```python
from build123d import *

# Parameters (mm, degrees)
F1_DEPTH = 25.4
F2_R     = 34.657222649
F3_DEPTH = 47.498
F4_R     = 5.08
F5_R     = 12.7
F6_DEPTH = 47.499
F7_R     = 5.08


with BuildPart() as f1:
    # F0 (on Top) → F1 (new body)
    with BuildSketch(Plane.XY):
        Polygon((43.3867163956, -75.1479971708), (43.3867163956, 75.1479971708), (-86.7734327912, 0), align=None)
    extrude(amount=F1_DEPTH)

    # F2 (on Top) → F3 (join)
    with BuildSketch(Plane.XY):
        Circle(F2_R)
    extrude(amount=F3_DEPTH)

    # F4
    f4_edges = [f1.edges().sort_by_distance(p)[0] for p in [
        (-34.657223, 0, 25.4),
        (-34.657223, 0, 47.498),
    ]]
    fillet(f4_edges, radius=F4_R)

    # F5 (on face) → F6 (cut, through all)
    with BuildSketch(Plane.XY.offset(47.498)):
        Circle(F5_R)
    extrude(amount=-F6_DEPTH, mode=Mode.SUBTRACT)

    # F7
    f7_edges = [f1.edges().sort_by_distance(p)[0] for p in [
        (43.386716, 0, 25.4),
        (-21.693358, -37.573999, 25.4),
        (-21.693358, 37.573999, 25.4),
        (43.386716, -75.147997, 12.7),
        (43.386716, 75.147997, 12.7),
        (-86.773433, 0, 12.7),
    ]]
    fillet(f7_edges, radius=F7_R)

    # F8 (on Right) → F9 (revolve)
    with BuildSketch(Plane.YZ):
        with BuildLine():
            Line((13.7427253649, 77.7795091271), (13.7427253649, 38.8897545636))
            add(Edge.make_bspline(
                [(13.7427253649, 77.7795091271), (19.7552349789, 72.2247905159), (30.7430265403, 62.0736067006), (63.7135258095, 65.9775971528), (32.8505351499, 49.2475903212), (13.7427253649, 38.8897545636)],
                knots=[0, 0, 0, 0, 0.3152034483, 0.5760306447, 1, 1, 1, 1], degree=3))
        make_face()
    revolve(axis=Axis((0, 0, 37.3068228364), (0, 0, 1)))


solid = f1.part
```
Model file for the job. Use its own axes, mm. A direction names the side the tool comes from. Give positions to 0.01 mm unless a question says otherwise; leave off trailing zeros. Loops run counter-clockwise (first coordinate to the right, second up) from the corner with the lowest first, then second, coordinate; pieces in that order, holes last. Notation, with made-up numbers: (-37, -18.75) -> (-27, -18.75) arc R23 cw to (-27, -1.75) -> close; hole circle Ø3 at (-38.75, -22). An arc over 180 degrees is marked (long way). Use CSV: the item, a comma, the result in double quotes. Start each with the question number.
1) Slice it at B-B on z = 28. Give the cut face in (x, y), plus the area to 3 significant figures.
2) Slice it at A-A on z = 18.5. Give the cut face in (x, y).
3) Wall check: line 1 (Y direction, x = 0, z = 33.5); line 2 (Z direction, x = -39, y = 11); line 3 (Y direction, x = 0, z = 17). Give the ranges that are in metal, low to high.
4) Mould opens along X. For faces 4 (the flat face through (9.1, -9.1, 47.498)), 5 (the flat face through (-51, 0, 25.4)), 6 (the cylindrical face through (12.038, 55.285, 23.951)), 7 (the cylindrical face through (-2.75, -12.4, 24.08)) say: released by +X, released by -X, zero draft, split by the parting line, or undercut.
5) Tool access for faces 1 (the flat face through (43.387, -1, 10)), 2 (the cylindrical face through (33.057, 10.41, 36.365)), 3 (the cylindrical face through (-54.57, 16.83, 23.95)): list every direction of +Z, -Z, +X, -X, +Y, -Y with a clear straight run to the whole face (end or side of a thin tool).
6) Flat gauge pins, fed straight in: pin 1 Ø2 at (x, z) = (-22.5, 37.5) entering from -Y; pin 2 Ø1 at (x, y) = (17.5, 55) entering from +Z; pin 3 Ø1.5 at (x, y) = (-48, 22) entering from +Z. Where does each tip first touch, or does it go through?
Computed values:
1,outline,"circle Ø70.61 at (0, 0); hole circle Ø25.4 at (0, 0)"
1,area,"3,410 mm^2"
2,outline,"(-79.15, -4.4) -> (35.77, -70.75) arc R5.08 ccw to (43.39, -66.35) -> (43.39, 66.35) arc R5.08 ccw to (35.77, 70.75) -> (-79.15, 4.4) arc R5.08 ccw to start; hole circle Ø25.4 at (0, 0)"
3,line 1,"y = -34.66 to -12.7, 12.7 to 34.66"
3,line 2,"z = 0 to 25.4, 53.91 to 64.01"
3,line 3,"y = -50.1 to -12.7, 12.7 to 50.1"
4,face 4,"undercut"
4,face 5,"zero draft"
4,face 6,"released by -X"
4,face 7,"undercut"
5,face 1,"-Z, +X, +Y, -Y"
5,face 2,"none"
5,face 3,"-X, +Y"
6,pin 1,"stops at y = -27.18"
6,pin 2,"stops at z = 25.4"
6,pin 3,"stops at z = 23.46"
